Here's how the part is built. I have some questions about the finished solid (model axes, mm). Face numbers are marked on the shaded views. A direction names the side the tool comes from. Coordinates: 2 decimals unless noted, no trailing zeros. Write each loop counter-clockwise with the first axis right and the second up, starting at its lowest first coordinate (ties: lowest second). Pieces come first, ordered by that corner, then holes.
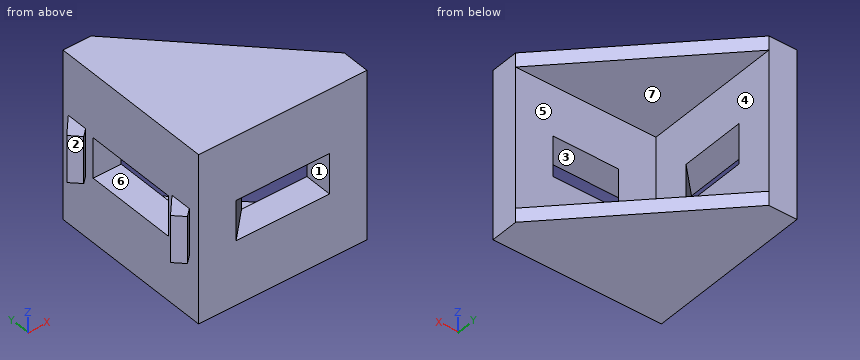
from build123d import *

# Parameters (mm, degrees)
BOSS_EXTRUDE1_DEPTH = 9
CUT_EXTRUDE1_DEPTH  = 7.5
CUT_EXTRUDE2_DEPTH  = 2.15
BOSS_EXTRUDE2_DEPTH = 2.5
SKETCH8_W           = 5
SKETCH8_H           = 2.300783428
SKETCH8_H_2         = 2.300783429
CUT_EXTRUDE6_DEPTH  = 2.54


with BuildPart() as part:
    # Sketch1 → Boss-Extrude1 (new, symmetric)
    with BuildSketch(Plane.XY):
        Polygon((0, 0), (0, 18), (3, 18), (18, 3), (18, 0), align=None)
    extrude(amount=BOSS_EXTRUDE1_DEPTH, both=True)

    # Sketch2 → Cut-Extrude1 (cut, symmetric)
    with BuildSketch(Plane.XY):
        Polygon((3, 18), (3, 3), (18, 3), align=None)
    extrude(amount=CUT_EXTRUDE1_DEPTH, both=True, mode=Mode.SUBTRACT)

    # Sketch3 → Cut-Extrude2 (cut, symmetric)
    with BuildSketch(Plane.XY):
        Polygon((0, 14), (3, 14), (3, 7), (0, 4), align=None)
        Polygon((7, 3), (14, 3), (14, 0), (4, 0), align=None)
    extrude(amount=CUT_EXTRUDE2_DEPTH, both=True, mode=Mode.SUBTRACT)

    # Sketch4 → Boss-Extrude2 (add, symmetric)
    with BuildSketch(Plane.XY):
        Polygon((1.504575227, -1.8), (0.511249685, -0.790946088), (1.234750477, 0), (3.535533906, 0), align=None)
        Polygon((0, 3.535533906), (-1.8, 1.504575227), (-0.790946088, 0.511249685), (0, 1.234750477), align=None)
        Polygon((0, 17.3), (0, 14.999216572), (-0.790946088, 14.275715779), (-1.8, 15.269041321), align=None)
        Polygon((14.999216572, 0), (14.275715779, -0.790946088), (15.269041321, -1.8), (17.3, 0), align=None)
    extrude(amount=BOSS_EXTRUDE2_DEPTH, both=True)

    # Sketch8 → Cut-Extrude6 (cut)
    with BuildSketch(Plane(origin=(114.3, 0, -271.000209725), x_dir=(0, 0, 1), z_dir=(0, 1, 0))):
        with Locations((271.000209725, -98.150391714)):
            Rectangle(SKETCH8_W, SKETCH8_H)
        with Locations((271.000209725, -111.914857809)):
            Rectangle(SKETCH8_W, SKETCH8_H_2)
    extrude(amount=-CUT_EXTRUDE6_DEPTH, mode=Mode.SUBTRACT)


with BuildPart() as cut_extrude6_kept_piece:
    # of the separate pieces the step leaves, the one the design keeps (cut_extrude6_pieces_kept)
    add(part.part.solids().sort_by_distance((0, 0, -9))[0])


solid = cut_extrude6_kept_piece.part
1. For pin 1 Ø0.9 at (x, y) = (-0.5, 15.5) entering from -Z; pin 2 Ø0.5 at (x, y) = (-1, 2.5) entering from +Z; pin 3 Ø3 at (y, z) = (8, 1.5) entering from +X, each with a flat end and sliding along its axis, tell me the tip position at first contact or that it passes through.
2. Thinking about a two-plate mould opening in Y: for the marked faces 5, 6 and 7, which applies, pulls with the +Y half, pulls with the -Y half, needs draft (parallel to the pull), parting line crosses it, or undercut?
3. I want a section at A-A (z = 1). List the corners of the cut face in (x, y) for me, then the cut area to 3 significant figures.
4. On a 3-axis mill with a long thin cutter (end or side, diameter ignored), from which of +Z, -Z, +X, -X, +Y, -Y can I reach the whole of each face in a straight line? I mean the marked faces 1, 2, 3 and 4. Say none if no direction works.
5. If I drill on line 1 (Z direction, x = 8.5, y = 1.75); line 2 (Z direction, x = 6.75, y = 13); line 3 (Y direction, x = 10.75, z = -3.5), over which ranges is the centre line in solid material (lowest first)?
6. I want a section at D-D (y = 5.5). List the corners of the cut face in (x, z) for me.
7. I want a section at C-C (x = 8.75). List the corners of the cut face in (y, z) for me, then the cut area to 4 significant figures.
8. I want a section at B-B (y = 11). List the corners of the cut face in (x, z) for me.
Response values:
1. pin 1: stops at z = -2.5
1. pin 2: stops at z = 2.5
1. pin 3: stops at x = 3
2. face 5: pulls with the +Y half
2. face 6: undercut
2. face 7: needs draft
3. outline: (-1.8, 1.5) - (-0.79, 0.51) - (0, 1.23) - (0, 0) - (4, 0) - (7, 3) - (3, 3) - (3, 7) - (0, 4) - (0, 3.54) - close; (-1.8, 15.27) - (-0.79, 14.28) - (0, 15) - (0, 14) - (3, 14) - (3, 18) - (0, 18) - (0, 17.3) - close; (14, 0) - (18, 0) - (18, 3) - (14, 3) - close
3. area: 53.7 mm2
4. face 1: +Y, -Y
4. face 2: +Z, -Z, -X
4. face 3: -Y
4. face 4: +X, +Y
5. line 1: z = -9 to -2.15, 2.15 to 9
5. line 2: z = -9 to -7.5, 7.5 to 9
5. line 3: y = 0 to 3
6. outline: (0, -9) - (15.5, -9) - (15.5, -7.5) - (3, -7.5) - (3, 7.5) - (15.5, 7.5) - (15.5, 9) - (0, 9) - (0, 2.15) - (1.5, 2.15) - (1.5, -2.15) - (0, -2.15) - close
7. outline: (0, -9) - (12.25, -9) - (12.25, -7.5) - (3, -7.5) - (3, -2.15) - (0, -2.15) - close; (0, 2.15) - (3, 2.15) - (3, 7.5) - (12.25, 7.5) - (12.25, 9) - (0, 9) - close
7. area: 68.85 mm2
8. outline: (0, -9) - (10, -9) - (10, -7.5) - (3, -7.5) - (3, -2.15) - (0, -2.15) - close; (0, 2.15) - (3, 2.15) - (3, 7.5) - (10, 7.5) - (10, 9) - (0, 9) - close
